Geometry: see drawing. Coordinates: mm, zero at the bounding-box minimum. A direction names the side the tool comes from. Coordinates: 2 decimals unless noted, no trailing zeros. Write each loop counter-clockwise with the first axis right and the second up, starting at its lowest first coordinate (ties: lowest second). Pieces come first, ordered by that corner, then holes. Notation, with made-up numbers: M -16.5,65.25 L 16.5,65.25 A28 cw 16.5,93.25 Z; hole C 60,2 d7. An arc over 180 degrees is marked long. Answer as CSV lines item,"result". Start each with the question number.
1. Section D-D on x = 111.95. Return the cut outline in (y, z), plus the area to 3 significant figures.
2. Mould query, pull axis Z, two halves, no side actions, for the marked faces 4, 5 and 6. Classes: pulls with the +Z half, pulls with the -Z half, needs draft (parallel to the pull), parting line crosses it, or undercut.
3. Contact query for flat-ended pins moving along their axis: pin 1 Ø6 at (y, z) = (15, 16.5) entering from +X; pin 2 Ø8 at (y, z) = (14, 23) entering from -X; pin 3 Ø7 at (x, y) = (38.5, 14) entering from +Z. Output: stop coordinate, or through.
4. Section C-C on y = 3. Return the cut outline in (x, z).
5. Section B-B on x = 19.5. Return the cut outline in (y, z).
6. Reachability of the marked faces 1, 2 and 3 from +Z, -Z, +X, -X, +Y, -Y: full face, straight path, thin tool, end or side. Return the list, or none.
7. Section A-A on y = 12. Return the cut outline in (x, z).
8. Line query: probe 1 along X at (y, z) = (12, 47.5); probe 2 along Y at (x, z) = (86.95, 45.25); probe 3 along Y at (x, z) = (41.5, 3). Output: solid intervals per line, ascending. Write a range as [from, to].
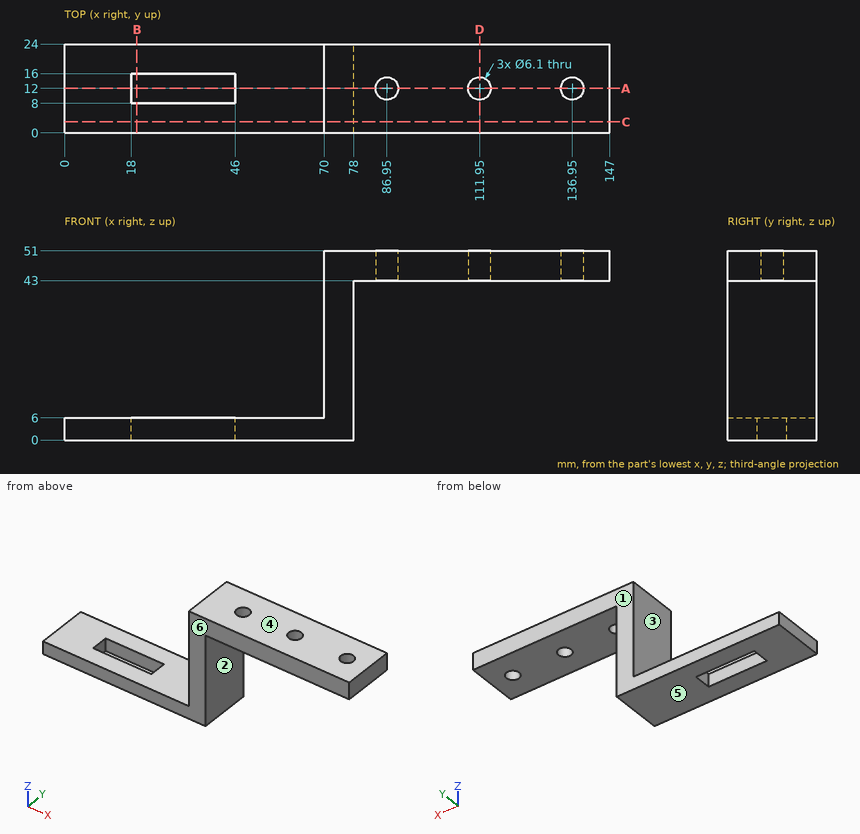
Values:
1,outline,"M 0,43 L 8.95,43 L 8.95,51 L 0,51 Z; M 15.05,43 L 24,43 L 24,51 L 15.05,51 Z"
1,area,"143 mm²"
2,face 4,"pulls with the +Z half"
2,face 5,"pulls with the -Z half"
2,face 6,"needs draft"
3,pin 1,"x = 78"
3,pin 2,"x = 70"
3,pin 3,"z = 6"
4,outline,"M 0,0 L 78,0 L 78,43 L 147,43 L 147,51 L 70,51 L 70,6 L 0,6 Z"
5,outline,"M 0,0 L 8,0 L 8,6 L 0,6 Z; M 16,0 L 24,0 L 24,6 L 16,6 Z"
6,face 1,"+Z, -Z, +X, -X, +Y"
6,face 2,"-Z, +X, +Y, -Y"
6,face 3,"+Z, -X, +Y, -Y"
7,outline,"M 0,0 L 18,0 L 18,6 L 0,6 Z; M 46,0 L 78,0 L 78,43 L 83.9,43 L 83.9,51 L 70,51 L 70,6 L 46,6 Z; M 90,43 L 108.9,43 L 108.9,51 L 90,51 Z; M 115,43 L 133.9,43 L 133.9,51 L 115,51 Z; M 140,43 L 147,43 L 147,51 L 140,51 Z"
8,probe 1,"[70, 83.9], [90, 108.9], [115, 133.9], [140, 147]"
8,probe 2,"[0, 8.95], [15.05, 24]"
8,probe 3,"[0, 8], [16, 24]"
